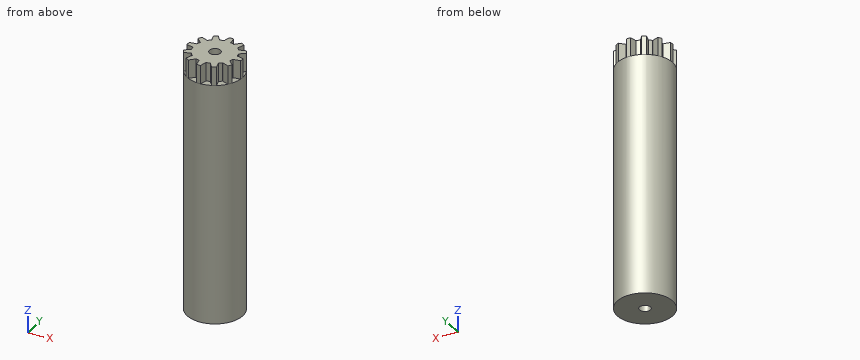
from build123d import *

# Parameters (mm, degrees)
SKETCH1_R           = 7.5
BOSS_EXTRUDE1_DEPTH = 65
BOSS_EXTRUDE7_DEPTH = 5
SKETCH5_R           = 1.5
CUT_EXTRUDE1_DEPTH  = 71.803359707


with BuildPart() as part:
    # Sketch1 → Boss-Extrude1 (new body)
    with BuildSketch(Plane.XY):
        Circle(SKETCH1_R)
    extrude(amount=BOSS_EXTRUDE1_DEPTH)

    # Sketch4 → Boss-Extrude7 (add)
    with BuildSketch(Plane.XY.offset(65)):
        with BuildLine():
            Line((1.29482372, 5.515672238), (1.312530063, 5.591097474))
            Line((1.312530063, 5.591097474), (1.052683226, 7.446710482))
            Line((1.052683226, 7.446710482), (-0.061368597, 7.52049685))
            Line((-0.061368597, 7.52049685), (-0.563675613, 5.715363149))
            Line((-0.563675613, 5.715363149), (-0.556071495, 5.63826154))
            ThreePointArc((-0.556071495, 5.63826154), (0.374427225, 5.653230311), (1.29482372, 5.515672238))
        make_face()
        with BuildLine():
            ThreePointArc((2.337558729, 5.160913474), (1.824832598, 5.363692263), (1.29482372, 5.515672238))
            Line((1.29482372, 5.515672238), (0, 0))
            Line((0, 0), (2.337558729, 5.160913474))
        make_face()
        with BuildLine():
            Line((0, 0), (1.29482372, 5.515672238))
            ThreePointArc((1.29482372, 5.515672238), (0.374427225, 5.653230311), (-0.556071495, 5.63826154))
            Line((-0.556071495, 5.63826154), (0, 0))
        make_face()
        with BuildLine():
            Line((-1.636485884, 5.424124137), (0, 0))
            Line((0, 0), (-0.556071495, 5.63826154))
            ThreePointArc((-0.556071495, 5.63826154), (-1.101494744, 5.557510057), (-1.636485884, 5.424124137))
        make_face()
        with BuildLine():
            Line((2.337558729, 5.160913474), (0, 0))
            Line((0, 0), (3.879186354, 4.129300417))
            ThreePointArc((3.879186354, 4.129300417), (3.150878645, 4.708627451), (2.337558729, 5.160913474))
        make_face()
        with BuildLine():
            Line((4.604841979, 3.300702811), (0, 0))
            Line((0, 0), (5.424124137, 1.636485884))
            ThreePointArc((5.424124137, 1.636485884), (5.083054676, 2.502351667), (4.604841979, 3.300702811))
        make_face()
        with BuildLine():
            Line((3.879186354, 4.129300417), (0, 0))
            Line((0, 0), (4.604841979, 3.300702811))
            ThreePointArc((4.604841979, 3.300702811), (4.262197519, 3.732677459), (3.879186354, 4.129300417))
        make_face()
        with BuildLine():
            Line((5.63826154, 0.556071495), (0, 0))
            Line((0, 0), (5.515672238, -1.29482372))
            ThreePointArc((5.515672238, -1.29482372), (5.628005488, -0.651738388), (5.665616357, 0))
            ThreePointArc((5.665616357, 0), (5.65877352, 0.27837196), (5.63826154, 0.556071495))
        make_face()
        with BuildLine():
            Line((5.424124137, 1.636485884), (0, 0))
            Line((0, 0), (5.63826154, 0.556071495))
            ThreePointArc((5.63826154, 0.556071495), (5.557510057, 1.101494744), (5.424124137, 1.636485884))
        make_face()
        with BuildLine():
            Line((5.160913474, -2.337558729), (0, 0))
            Line((0, 0), (4.129300417, -3.879186354))
            ThreePointArc((4.129300417, -3.879186354), (4.708627451, -3.150878645), (5.160913474, -2.337558729))
        make_face()
        with BuildLine():
            Line((5.515672238, -1.29482372), (0, 0))
            Line((0, 0), (5.160913474, -2.337558729))
            ThreePointArc((5.160913474, -2.337558729), (5.363692263, -1.824832598), (5.515672238, -1.29482372))
        make_face()
        with BuildLine():
            Line((3.300702811, -4.604841979), (0, 0))
            Line((0, 0), (1.636485884, -5.424124137))
            ThreePointArc((1.636485884, -5.424124137), (2.502351667, -5.083054676), (3.300702811, -4.604841979))
        make_face()
        with BuildLine():
            Line((4.129300417, -3.879186354), (0, 0))
            Line((0, 0), (3.300702811, -4.604841979))
            ThreePointArc((3.300702811, -4.604841979), (3.732677459, -4.262197519), (4.129300417, -3.879186354))
        make_face()
        with BuildLine():
            Line((0.556071495, -5.63826154), (0, 0))
            Line((0, 0), (-1.29482372, -5.515672238))
            ThreePointArc((-1.29482372, -5.515672238), (-0.374427225, -5.653230311), (0.556071495, -5.63826154))
        make_face()
        with BuildLine():
            Line((1.636485884, -5.424124137), (0, 0))
            Line((0, 0), (0.556071495, -5.63826154))
            ThreePointArc((0.556071495, -5.63826154), (1.101494744, -5.557510057), (1.636485884, -5.424124137))
        make_face()
        with BuildLine():
            Line((-2.337558729, -5.160913474), (0, 0))
            Line((0, 0), (-3.879186354, -4.129300417))
            ThreePointArc((-3.879186354, -4.129300417), (-3.150878645, -4.708627451), (-2.337558729, -5.160913474))
        make_face()
        with BuildLine():
            Line((-1.29482372, -5.515672238), (0, 0))
            Line((0, 0), (-2.337558729, -5.160913474))
            ThreePointArc((-2.337558729, -5.160913474), (-1.824832598, -5.363692263), (-1.29482372, -5.515672238))
        make_face()
        with BuildLine():
            Line((-4.604841979, -3.300702811), (0, 0))
            Line((0, 0), (-5.424124137, -1.636485884))
            ThreePointArc((-5.424124137, -1.636485884), (-5.083054676, -2.502351667), (-4.604841979, -3.300702811))
        make_face()
        with BuildLine():
            Line((-3.879186354, -4.129300417), (0, 0))
            Line((0, 0), (-4.604841979, -3.300702811))
            ThreePointArc((-4.604841979, -3.300702811), (-4.262197519, -3.732677459), (-3.879186354, -4.129300417))
        make_face()
        with BuildLine():
            Line((-5.63826154, -0.556071495), (0, 0))
            Line((0, 0), (-5.515672238, 1.29482372))
            ThreePointArc((-5.515672238, 1.29482372), (-5.653230311, 0.374427225), (-5.63826154, -0.556071495))
        make_face()
        with BuildLine():
            Line((-5.424124137, -1.636485884), (0, 0))
            Line((0, 0), (-5.63826154, -0.556071495))
            ThreePointArc((-5.63826154, -0.556071495), (-5.557510057, -1.101494744), (-5.424124137, -1.636485884))
        make_face()
        with BuildLine():
            Line((-5.160913474, 2.337558729), (0, 0))
            Line((0, 0), (-4.129300417, 3.879186354))
            ThreePointArc((-4.129300417, 3.879186354), (-4.708627451, 3.150878645), (-5.160913474, 2.337558729))
        make_face()
        with BuildLine():
            Line((-5.515672238, 1.29482372), (0, 0))
            Line((0, 0), (-5.160913474, 2.337558729))
            ThreePointArc((-5.160913474, 2.337558729), (-5.363692263, 1.824832598), (-5.515672238, 1.29482372))
        make_face()
        with BuildLine():
            Line((-3.300702811, 4.604841979), (0, 0))
            Line((0, 0), (-1.636485884, 5.424124137))
            ThreePointArc((-1.636485884, 5.424124137), (-2.502351667, 5.083054676), (-3.300702811, 4.604841979))
        make_face()
        with BuildLine():
            Line((-4.129300417, 3.879186354), (0, 0))
            Line((0, 0), (-3.300702811, 4.604841979))
            ThreePointArc((-3.300702811, 4.604841979), (-3.732677459, 4.262197519), (-4.129300417, 3.879186354))
        make_face()
        with BuildLine():
            Line((2.369524174, 5.231487486), (2.337558729, 5.160913474))
            ThreePointArc((2.337558729, 5.160913474), (3.150878645, 4.708627451), (3.879186354, 4.129300417))
            Line((3.879186354, 4.129300417), (3.932233115, 4.185767416))
            Line((3.932233115, 4.185767416), (4.635005657, 5.922698839))
            Line((4.635005657, 5.922698839), (3.707101661, 6.54362562))
            Line((3.707101661, 6.54362562), (2.369524174, 5.231487486))
        make_face()
        with BuildLine():
            ThreePointArc((4.604841979, 3.300702811), (5.083054676, 2.502351667), (5.424124137, 1.636485884))
            Line((5.424124137, 1.636485884), (5.498297479, 1.658864359))
            Line((5.498297479, 1.658864359), (6.975382065, 2.811704825))
            Line((6.975382065, 2.811704825), (6.482257022, 3.813395189))
            Line((6.482257022, 3.813395189), (4.667811873, 3.345838975))
            Line((4.667811873, 3.345838975), (4.604841979, 3.300702811))
        make_face()
        with BuildLine():
            ThreePointArc((5.665616357, 0), (5.628005488, -0.651738388), (5.515672238, -1.29482372))
            Line((5.515672238, -1.29482372), (5.591097474, -1.312530063))
            Line((5.591097474, -1.312530063), (7.446710482, -1.052683226))
            Line((7.446710482, -1.052683226), (7.52049685, 0.061368597))
            Line((7.52049685, 0.061368597), (5.715363149, 0.563675613))
            Line((5.715363149, 0.563675613), (5.63826154, 0.556071495))
            ThreePointArc((5.63826154, 0.556071495), (5.65877352, 0.27837196), (5.665616357, 0))
        make_face()
        with BuildLine():
            ThreePointArc((5.160913474, -2.337558729), (4.708627451, -3.150878645), (4.129300417, -3.879186354))
            Line((4.129300417, -3.879186354), (4.185767416, -3.932233115))
            Line((4.185767416, -3.932233115), (5.922698839, -4.635005657))
            Line((5.922698839, -4.635005657), (6.54362562, -3.707101661))
            Line((6.54362562, -3.707101661), (5.231487486, -2.369524174))
            Line((5.231487486, -2.369524174), (5.160913474, -2.337558729))
        make_face()
        with BuildLine():
            ThreePointArc((3.300702811, -4.604841979), (2.502351667, -5.083054676), (1.636485884, -5.424124137))
            Line((1.636485884, -5.424124137), (1.658864359, -5.498297479))
            Line((1.658864359, -5.498297479), (2.811704825, -6.975382065))
            Line((2.811704825, -6.975382065), (3.813395189, -6.482257022))
            Line((3.813395189, -6.482257022), (3.345838975, -4.667811873))
            Line((3.345838975, -4.667811873), (3.300702811, -4.604841979))
        make_face()
        with BuildLine():
            ThreePointArc((0.556071495, -5.63826154), (-0.374427225, -5.653230311), (-1.29482372, -5.515672238))
            Line((-1.29482372, -5.515672238), (-1.312530063, -5.591097474))
            Line((-1.312530063, -5.591097474), (-1.052683226, -7.446710482))
            Line((-1.052683226, -7.446710482), (0.061368597, -7.52049685))
            Line((0.061368597, -7.52049685), (0.563675613, -5.715363149))
            Line((0.563675613, -5.715363149), (0.556071495, -5.63826154))
        make_face()
        with BuildLine():
            ThreePointArc((-2.337558729, -5.160913474), (-3.150878645, -4.708627451), (-3.879186354, -4.129300417))
            Line((-3.879186354, -4.129300417), (-3.932233115, -4.185767416))
            Line((-3.932233115, -4.185767416), (-4.635005657, -5.922698839))
            Line((-4.635005657, -5.922698839), (-3.707101661, -6.54362562))
            Line((-3.707101661, -6.54362562), (-2.369524174, -5.231487486))
            Line((-2.369524174, -5.231487486), (-2.337558729, -5.160913474))
        make_face()
        with BuildLine():
            ThreePointArc((-4.604841979, -3.300702811), (-5.083054676, -2.502351667), (-5.424124137, -1.636485884))
            Line((-5.424124137, -1.636485884), (-5.498297479, -1.658864359))
            Line((-5.498297479, -1.658864359), (-6.975382065, -2.811704825))
            Line((-6.975382065, -2.811704825), (-6.482257022, -3.813395189))
            Line((-6.482257022, -3.813395189), (-4.667811873, -3.345838975))
            Line((-4.667811873, -3.345838975), (-4.604841979, -3.300702811))
        make_face()
        with BuildLine():
            ThreePointArc((-5.63826154, -0.556071495), (-5.653230311, 0.374427225), (-5.515672238, 1.29482372))
            Line((-5.515672238, 1.29482372), (-5.591097474, 1.312530063))
            Line((-5.591097474, 1.312530063), (-7.446710482, 1.052683226))
            Line((-7.446710482, 1.052683226), (-7.52049685, -0.061368597))
            Line((-7.52049685, -0.061368597), (-5.715363149, -0.563675613))
            Line((-5.715363149, -0.563675613), (-5.63826154, -0.556071495))
        make_face()
        with BuildLine():
            ThreePointArc((-5.160913474, 2.337558729), (-4.708627451, 3.150878645), (-4.129300417, 3.879186354))
            Line((-4.129300417, 3.879186354), (-4.185767416, 3.932233115))
            Line((-4.185767416, 3.932233115), (-5.922698839, 4.635005657))
            Line((-5.922698839, 4.635005657), (-6.54362562, 3.707101661))
            Line((-6.54362562, 3.707101661), (-5.231487486, 2.369524174))
            Line((-5.231487486, 2.369524174), (-5.160913474, 2.337558729))
        make_face()
        with BuildLine():
            ThreePointArc((-3.300702811, 4.604841979), (-2.502351667, 5.083054676), (-1.636485884, 5.424124137))
            Line((-1.636485884, 5.424124137), (-1.658864359, 5.498297479))
            Line((-1.658864359, 5.498297479), (-2.811704825, 6.975382065))
            Line((-2.811704825, 6.975382065), (-3.813395189, 6.482257022))
            Line((-3.813395189, 6.482257022), (-3.345838975, 4.667811873))
            Line((-3.345838975, 4.667811873), (-3.300702811, 4.604841979))
        make_face()
    extrude(amount=BOSS_EXTRUDE7_DEPTH)

    # Sketch5 → Cut-Extrude1 (cut, through all)
    with BuildSketch(Plane(origin=(0, 0, 0), x_dir=(-1, 0, 0), z_dir=(0, 0, -1))):
        Circle(SKETCH5_R)
    extrude(amount=-CUT_EXTRUDE1_DEPTH, mode=Mode.SUBTRACT)


solid = part.part
Could you check a few things on this model? Use its own coordinates, in mm. Coordinates: 2 decimals unless noted, no trailing zeros. Order: outer loops, then holes, each group sorted by start corner. A loop starts at its lowest first (then second) coordinate and runs counter-clockwise, first axis right, second up. Notation, with made-up numbers: (54.25, 72.5) - (102.25, 72.5) arc R18 ccw to (102.25, 104.5) - close; hole circle Ø4 at (-4.5, 68). An arc over 180 degrees is marked (long way). Answer in a Markdown table with one row per item. Add a question column.
(1) If we section it at A-A, the plane z = 28.5: Please give me the cut outline in (x, y).
(2) Will these pins go through, and if not, where does the flat tip stop? pin 1 (8 mm diameter, centred on y = -3, z = 23, fed in from +X); pin 2 (4 mm diameter, centred on y = -2.5, z = 50.5, fed in from -X); pin 3 (5 mm diameter, centred on x = -4, z = 43.5, fed in from -Y).
(3) I need wall thicknesses on L1, parallel to Y at x = 0, z = 30; L2, parallel to Y at x = 1, z = 39; L3, parallel to Y at x = -2.75, z = 5. Which ranges of each line are inside material? Lowest first, please.
Results are:
| question | item | result |
|---|---|---|
| 1 | outline | circle Ø15 at (0, 0); hole circle Ø3 at (0, 0) |
| 2 | pin 1 | stops at x = 7.5 |
| 2 | pin 2 | stops at x = -7.48 |
| 2 | pin 3 | stops at y = -7.35 |
| 3 | L1 | y = -7.5 to -1.5, 1.5 to 7.5 |
| 3 | L2 | y = -7.43 to -1.12, 1.12 to 7.43 |
| 3 | L3 | y = -6.98 to 6.98 |
